Source: three-view drawing plus pictorial views. Frame: mm from the lowest corner of the part. Give positions to 0.01 mm unless a question says otherwise; leave off trailing zeros. Order: outer loops, then holes, each group sorted by start corner. A loop starts at its lowest first (then second) coordinate and runs counter-clockwise, first axis right, second up. Notation, with made-up numbers: M -29,-35 L -8,-35 A22 cw -8,-4 Z; hole C 54.5,49.25 d2. An arc over 180 degrees is marked long. Use CSV: the item, a comma, the result in double quotes.
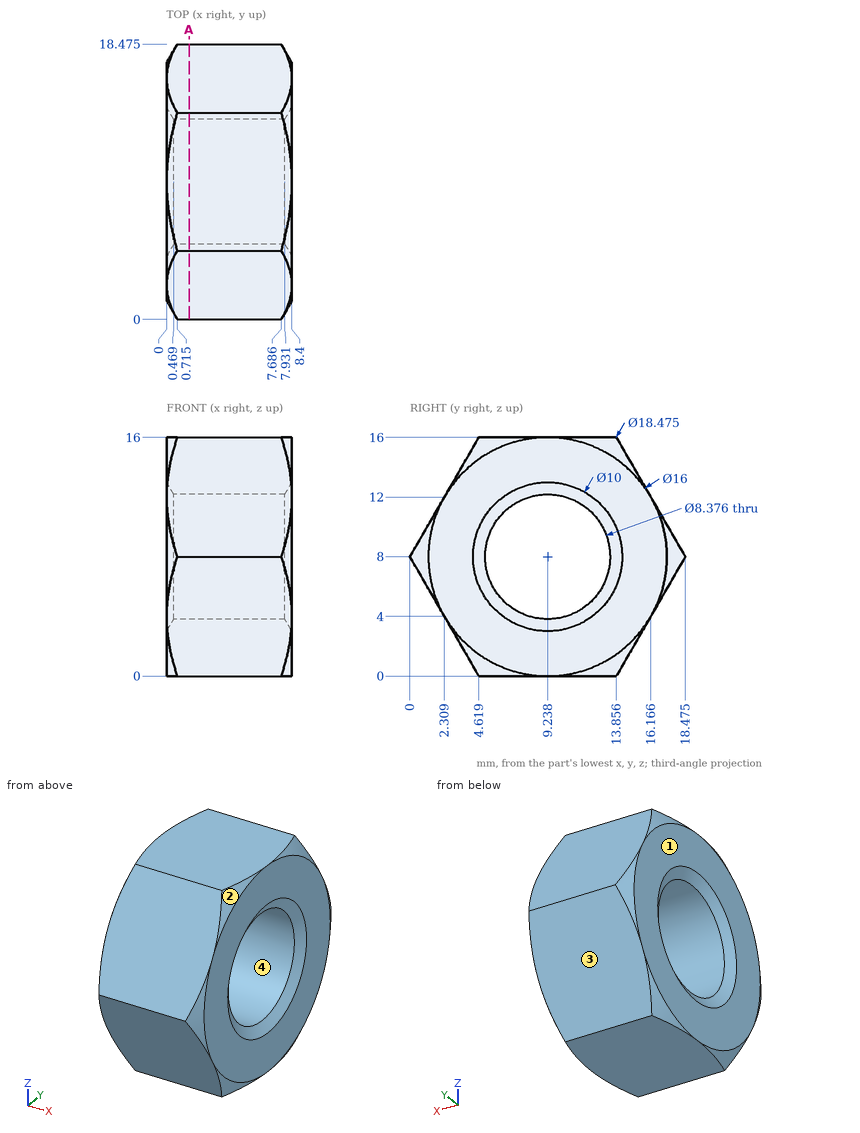
1. Pin query (flat end, axial travel): pin 1 Ø2 at (x, z) = (2, 14) entering from +Y. Return the tip coordinate at first contact, or that it passes through.
Answer:
pin 1,"y = 15.59"
2. Pull-direction query (Z, two-part tool) for the marked faces 1, 2, 3 and 4; classes: +Z half, -Z half, draft (parallel to the pull), parting line (faces both ways), or undercut.
Answer:
face 1,"draft"
face 2,"+Z half"
face 3,"-Z half"
face 4,"undercut"
3. Line query: line 1 (Z direction, x = 4.5, y = 8); line 2 (Z direction, x = 5, y = 8.5); line 3 (Y direction, x = 7.5, z = 11.75) (1 decimal). Output: solid intervals per line, ascending.
Answer:
line 1,"0 to 4, 12 to 16"
line 2,"0 to 3.88, 12.12 to 16"
line 3,"2.2 to 7.4, 11.1 to 16.3"
4. Section A-A, the plane x = 1.5. Return the cut outline in (y, z) (1 decimal).
Answer:
outline,"M 0,8 L 4.6,0 L 13.9,0 L 18.5,8 L 13.9,16 L 4.6,16 Z; hole C 9.2,8 d8.4"
